Geometry: final body of the model. Coordinates: model frame, mm. A direction names the side the tool comes from. Coordinates: 2 decimals unless noted, no trailing zeros. Write each loop counter-clockwise with the first axis right and the second up, starting at its lowest first coordinate (ties: lowest second). Pieces come first, ordered by that corner, then holes.
from build123d import *

# Parameters (mm, degrees)
SKETCH_1_W          = 15.8
SKETCH_1_H          = 7.8
EXTRUDE_1_DEPTH     = 9.6
SKETCH_2_W          = 15.8
SKETCH_2_H          = 6.199999898
CUT_EXTRUDE_1_DEPTH = 7.6
SKETCH_3_R          = 2.5
CUT_EXTRUDE_2_DEPTH = 1.8


with BuildPart() as part:
    # Эскиз1 → Бобышка-Вытянуть1 (new body)
    with BuildSketch(Plane(origin=(0, 0, 0), x_dir=(1, 0, 0), z_dir=(0, 1, 0))):
        Rectangle(SKETCH_1_W, SKETCH_1_H)
    extrude(amount=EXTRUDE_1_DEPTH)

    # Эскиз2 → Вырез-Вытянуть1 (cut)
    with BuildSketch(Plane(origin=(0, 9.6, 0), x_dir=(1, 0, 0), z_dir=(0, 1, 0))):
        with Locations((0, -0.800000051)):
            Rectangle(SKETCH_2_W, SKETCH_2_H)
    extrude(amount=-CUT_EXTRUDE_1_DEPTH, mode=Mode.SUBTRACT)

    # Эскиз3 → Вырез-Вытянуть2 (cut)
    with BuildSketch(Plane.XZ):
        with Locations(Location((-4, -7.4e-08, 0), (0, 0, 270))):
            Circle(SKETCH_3_R)
        with Locations(Location((3.874, -7.4e-08, 0), (0, 0, 270))):
            Circle(SKETCH_3_R)
    extrude(amount=-CUT_EXTRUDE_2_DEPTH, mode=Mode.SUBTRACT)


solid = part.part
Item 1: Pin query (flat end, axial travel): pin 1 (1.5 mm diameter, centred on x = 3.5, z = 0.5, fed in from -Y); pin 2 (1 mm diameter, centred on x = 1.5, z = 3, fed in from +Y); pin 3 (2.5 mm diameter, centred on x = -3, y = 7, fed in from +Z). Return the tip coordinate at first contact, or that it passes through.
Derived:
pin 1: stops at y = 1.8
pin 2: stops at y = 2
pin 3: stops at z = -2.3
Item 2: Set-up query: faces 1 (the flat face through (0, 6, -2.3)), 2 (the flat face through (0, 9.6, -3)), 3 (the cylindrical face through (1.433, 0.887, 0.542)). Return all of +Z, -Z, +X, -X, +Y, -Y with unobstructed straight access to the full face (end or side cutting, diameter ignored); none if empty.
Derived:
face 1: +Z, +X, -X, +Y
face 2: +Z, -Z, +X, -X, +Y
face 3: -Y
Item 3: Section A-A, the plane z = 0. Output: boundary loops of the cut face in (x, y).
Derived:
outline: (-7.9, 0) - (-6.5, 0) - (-6.5, 1.8) - (-1.5, 1.8) - (-1.5, 0) - (1.37, 0) - (1.37, 1.8) - (6.37, 1.8) - (6.37, 0) - (7.9, 0) - (7.9, 2) - (-7.9, 2) - close
Item 4: Material intervals for probe 1 along X at (y, z) = (0.4, 0); probe 2 along Z at (x, y) = (-6.5, 2.5); probe 3 along Y at (x, z) = (2.25, -1), sorted ascending.
Derived:
probe 1: x = -7.9 to -6.5, -1.5 to 1.37, 6.37 to 7.9
probe 2: z = -3.9 to -2.3
probe 3: y = 1.8 to 2
Item 5: Section C-C, the plane y = 1.5. Output: boundary loops of the cut face in (x, z), plus the area to 3 significant figures.
Derived:
outline: (-7.9, -3.9) - (7.9, -3.9) - (7.9, 3.9) - (-7.9, 3.9) - close; hole circle Ø5 at (-4, 0); hole circle Ø5 at (3.87, 0)
area: 84.0 mm2
Item 6: Section D-D, the plane y = 8.75. Output: boundary loops of the cut face in (x, z), plus the area to 3 significant figures.
Derived:
outline: (-7.9, -3.9) - (7.9, -3.9) - (7.9, -2.3) - (-7.9, -2.3) - close
area: 25.3 mm2
Item 7: Section B-B, the plane x = -0.25. Output: boundary loops of the cut face in (y, z), plus the area to 3 significant figures.
Derived:
outline: (0, -3.9) - (9.6, -3.9) - (9.6, -2.3) - (2, -2.3) - (2, 3.9) - (0, 3.9) - close
area: 27.8 mm2
Item 8: Pull-direction query (Z, two-part tool) for faces 4 (the flat face through (0, 1, 3.9)), 5 (the flat face through (-4, 1.8, 0)), 6 (the flat face through (0, 0, 0)); classes: released by +Z, released by -Z, zero draft, split by the parting line, or undercut.
Derived:
face 4: released by +Z
face 5: undercut
face 6: zero draft
